```python
from build123d import *

# Parameters (mm, degrees)
SKETCH1_R                 = 9.8
BOSS_EXTRUDE1_DEPTH       = 15.7
FILLET1_R                 = 1
SKETCH3_W                 = 41.9
SKETCH3_H                 = 37
BOSS_EXTRUDE2_DEPTH       = 37.89
SKETCH2_R                 = 1.55
CUT_EXTRUDE1_DEPTH        = 61.440388814
SKETCH4_W                 = 4.95
SKETCH4_H                 = 37
BOSS_EXTRUDE3_DEPTH       = 14.25
CUT_EXTRUDE_START         = -14.25
CUT_EXTRUDE_2_OUTLINE_W   = 1.15
CUT_EXTRUDE_2_OUTLINE_H   = 14.2
CUT_EXTRUDE_2_OUTLINE_W_2 = 1.900000227
CUT_EXTRUDE_2_OUTLINE_H_2 = 18.6
CUT_EXTRUDE_2_DEPTH       = 14.25
CUT_EXTRUDE_1_REACH       = 83.854
SKETCH_1_R                = 1.05
CUT_EXTRUDE3_START        = -5
SKETCH6_R                 = 1.41
CUT_EXTRUDE3_DEPTH        = 69.371779997
FILLET5_R                 = 2
MOVE_START                = 11.2
MOVE_FACE_1_OUTLINE_R     = 9.8
MOVE_FACE_1_DEPTH         = 4.5
SKETCH_4_R                = 11.200313663
CUT_EXTRUDE_3_DEPTH       = 38.09
SKETCH_6_W                = 2.268388773
SKETCH_6_H                = 19.352707125
EXTRUDE_1_DEPTH           = 5
CUT_EXTRUDE2_REACH        = 83.854
SKETCH5_R                 = 1.05
SKETCH_7_W                = 33.485055755
SKETCH_7_H                = 15.84059592
EXTRUDE_2_DEPTH           = 5.9
SKETCH_8_W                = 34.098293505
SKETCH_8_H                = 15.557673108
EXTRUDE_3_DEPTH           = 5.9
OTHER_START               = 11.2
OTHER_1_DEPTH             = 42.39
SKETCH_9_R                = 3.5
CUT_EXTRUDE_4_DEPTH       = 5


# Read off the part's stored shape, not the designer's step: 切除-拉伸2, 移动面1, 填充阵列1
with BuildPart() as part:
    # Sketch1 → Boss-Extrude1 (new body)
    with BuildSketch(Plane(origin=(0, 0, 0), x_dir=(1, 0, 0), z_dir=(0, 1, 0))):
        with Locations(Location((0, 0, 0), (0, 0, 270))):
            Circle(SKETCH1_R)
    extrude(amount=BOSS_EXTRUDE1_DEPTH)

    # Fillet1
    fillet1_edges = [part.edges().sort_by_distance(p)[0] for p in [
        (0, 0, -9.8),
    ]]
    fillet(fillet1_edges, radius=FILLET1_R)

    # Sketch3 → Boss-Extrude2 (add)
    with BuildSketch(Plane(origin=(0, 15.7, 0), x_dir=(1, 0, 0), z_dir=(0, 1, 0))):
        Rectangle(SKETCH3_W, SKETCH3_H)
    extrude(amount=BOSS_EXTRUDE2_DEPTH)

    # Sketch2 → Cut-Extrude1 (cut, through all)
    with BuildSketch(Plane(origin=(0, 0, 0), x_dir=(-1, 0, 0), z_dir=(0, -1, 0))):
        with Locations(Location((0, 6.999998127, 0), (0, 0, 90))):
            Circle(SKETCH2_R)
        with Locations(Location((6.999998127, 0, 0), (0, 0, 90))):
            Circle(SKETCH2_R)
        with Locations(Location((0, -6.999998127, 0), (0, 0, 90))):
            Circle(SKETCH2_R)
        with Locations(Location((-6.999998127, 0, 0), (0, 0, 90))):
            Circle(SKETCH2_R)
    extrude(amount=-CUT_EXTRUDE1_DEPTH, mode=Mode.SUBTRACT)

    # Sketch4 → Boss-Extrude3 (add)
    with BuildSketch(Plane(origin=(0, 53.59, 0), x_dir=(1, 0, 0), z_dir=(0, 1, 0))):
        with Locations((-18.475, 0)):
            Rectangle(SKETCH4_W, SKETCH4_H)
        with Locations((18.475, 0)):
            Rectangle(SKETCH4_W, SKETCH4_H)
    extrude(amount=BOSS_EXTRUDE3_DEPTH)

    # 切除-拉伸2 outline → 切除-拉伸2 (cut)
    with BuildSketch(Plane(origin=(0, 67.84, 0), x_dir=(1, 0, 0), z_dir=(0, 1, 0)).offset(CUT_EXTRUDE_START)):
        with Locations((16.575, 0)):
            Rectangle(CUT_EXTRUDE_2_OUTLINE_W, CUT_EXTRUDE_2_OUTLINE_H)
        with Locations((-16.950000113, 0)):
            Rectangle(CUT_EXTRUDE_2_OUTLINE_W_2, CUT_EXTRUDE_2_OUTLINE_H_2)
    extrude(amount=CUT_EXTRUDE_2_DEPTH, mode=Mode.SUBTRACT)

    # 草图1 → 切除-拉伸1 (cut, up to next)
    with BuildSketch(Plane(origin=(20.95, 0, 0), x_dir=(0, 0, -1), z_dir=(1, 0, 0)), mode=Mode.PRIVATE) as cut_extrude_1_sk1:
        with Locations((-10.25, 59.7)):
            Circle(SKETCH_1_R)
    cut_extrude_1_tool1 = extrude(cut_extrude_1_sk1.sketch, amount=-CUT_EXTRUDE_1_REACH, mode=Mode.PRIVATE) & part.part
    # 草图1 → 切除-拉伸1 (cut, up to next)
    with BuildSketch(Plane(origin=(20.95, 0, 0), x_dir=(0, 0, -1), z_dir=(1, 0, 0)), mode=Mode.PRIVATE) as cut_extrude_1_sk2:
        with Locations((10.25, 59.7)):
            Circle(SKETCH_1_R)
    cut_extrude_1_tool2 = extrude(cut_extrude_1_sk2.sketch, amount=-CUT_EXTRUDE_1_REACH, mode=Mode.PRIVATE) & part.part
    add(cut_extrude_1_tool1.solids().sort_by_distance((20.95, 59.7, 10.25))[0], mode=Mode.SUBTRACT)
    add(cut_extrude_1_tool2.solids().sort_by_distance((20.95, 59.7, -10.25))[0], mode=Mode.SUBTRACT)

    # Sketch6 → Cut-Extrude3 (cut, through all)
    with BuildSketch(Plane.XZ.offset(CUT_EXTRUDE3_START)):
        with Locations((0, 6.999998127)):
            Circle(SKETCH6_R)
        with Locations((0, -6.999998127)):
            Circle(SKETCH6_R)
        with Locations((-6.999998127, 0)):
            Circle(SKETCH6_R)
        with Locations((6.999998127, 0)):
            Circle(SKETCH6_R)
    extrude(amount=-CUT_EXTRUDE3_DEPTH, mode=Mode.SUBTRACT)

    # Fillet5
    fillet5_edges = [part.edges().sort_by_distance(p)[0] for p in [
        (20.95, 41.77, -18.5),
        (-20.95, 41.77, -18.5),
        (-20.95, 41.77, 18.5),
        (20.95, 41.77, 18.5),
    ]]
    fillet(fillet5_edges, radius=FILLET5_R)

    # Move Face 1 outline → Move Face 1 (add)
    with BuildSketch(Plane(origin=(0, 0, 0), x_dir=(1, 0, 0), z_dir=(0, 1, 0)).offset(MOVE_START)):
        with BuildLine():
            Line((20.95, -16.5), (20.95, 16.5))
            ThreePointArc((20.95, 16.5), (20.364213562, 17.914213562), (18.95, 18.5))
            Line((18.95, 18.5), (-18.95, 18.5))
            ThreePointArc((-18.95, 18.5), (-20.364213562, 17.914213562), (-20.95, 16.5))
            Line((-20.95, 16.5), (-20.95, -16.5))
            ThreePointArc((-20.95, -16.5), (-20.364213562, -17.914213562), (-18.95, -18.5))
            Line((-18.95, -18.5), (18.95, -18.5))
            ThreePointArc((18.95, -18.5), (20.364213562, -17.914213562), (20.95, -16.5))
        make_face()
        Circle(MOVE_FACE_1_OUTLINE_R, mode=Mode.SUBTRACT)
    extrude(amount=MOVE_FACE_1_DEPTH)

    # 草图4 → 切除-拉伸3 (cut)
    with BuildSketch(Plane(origin=(0, 53.59, 0), x_dir=(1, 0, 0), z_dir=(0, 1, 0))):
        with Locations(Location((0, 0, 0), (0, 0, 270))):
            Circle(SKETCH_4_R)
    extrude(amount=-CUT_EXTRUDE_3_DEPTH, mode=Mode.SUBTRACT)

    # 草图6 → 凸台-拉伸1 (add)
    with BuildSketch(Plane(origin=(0, 53.59, 0), x_dir=(1, 0, 0), z_dir=(0, 1, 0))):
        with Locations((-17.13419541, 0.070716348)):
            Rectangle(SKETCH_6_W, SKETCH_6_H)
    extrude(amount=EXTRUDE_1_DEPTH)

    # Sketch5 → Cut-Extrude2 (cut, up to next)
    with BuildSketch(Plane.ZY.offset(20.95), mode=Mode.PRIVATE) as cut_extrude2_sk1:
        with Locations((-10.25, 55.95)):
            Circle(SKETCH5_R)
    cut_extrude2_tool1 = extrude(cut_extrude2_sk1.sketch, amount=-CUT_EXTRUDE2_REACH, mode=Mode.PRIVATE) & part.part
    # Sketch5 → Cut-Extrude2 (cut, up to next)
    with BuildSketch(Plane.ZY.offset(20.95), mode=Mode.PRIVATE) as cut_extrude2_sk2:
        with Locations((10.25, 55.95)):
            Circle(SKETCH5_R)
    cut_extrude2_tool2 = extrude(cut_extrude2_sk2.sketch, amount=-CUT_EXTRUDE2_REACH, mode=Mode.PRIVATE) & part.part
    add(cut_extrude2_tool1.solids().sort_by_distance((-20.95, 55.95, -10.25))[0], mode=Mode.SUBTRACT)
    add(cut_extrude2_tool2.solids().sort_by_distance((-20.95, 55.95, 10.25))[0], mode=Mode.SUBTRACT)

    # 草图7 → 凸台-拉伸2 (add)
    with BuildSketch(Plane.XY.offset(18.5)):
        with Locations((0.159698038, 59.91970204)):
            Rectangle(SKETCH_7_W, SKETCH_7_H)
    extrude(amount=-EXTRUDE_2_DEPTH)

    # 草图8 → 凸台-拉伸3 (add)
    with BuildSketch(Plane(origin=(0, 0, -18.5), x_dir=(-1, 0, 0), z_dir=(0, 0, -1))):
        with Locations((-0.100853247, 60.061163446)):
            Rectangle(SKETCH_8_W, SKETCH_8_H)
    extrude(amount=-EXTRUDE_3_DEPTH)

    # Other 1 outline → Other 1 (cut)
    with BuildSketch(Plane(origin=(0, 0, 0), x_dir=(1, 0, 0), z_dir=(0, 1, 0)).offset(OTHER_START)):
        Polygon((15.149306373, -4.606205589), (16.015331777, -4.106205589), (16.015331777, -3.106205589), (15.149306373, -2.606205589), (14.283280969, -3.106205589), (14.283280969, -4.106205589), align=None)
        Polygon((16.015331777, 3.106205589), (16.015331777, 4.106205589), (15.149306373, 4.606205589), (14.283280969, 4.106205589), (14.283280969, 3.106205589), (15.149306373, 2.606205589), align=None)
        Polygon((-11.917262605, 6.212411178), (-11.051237202, 6.712411178), (-11.051237202, 7.712411178), (-11.917262605, 8.212411178), (-12.783288009, 7.712411178), (-12.783288009, 6.712411178), align=None)
        Polygon((-11.051237202, -7.712411178), (-11.051237202, -6.712411178), (-11.917262605, -6.212411178), (-12.783288009, -6.712411178), (-12.783288009, -7.712411178), (-11.917262605, -8.212411178), align=None)
        Polygon((13.933288009, -6.712411178), (13.067262605, -6.212411178), (12.201237202, -6.712411178), (12.201237202, -7.712411178), (13.067262605, -8.212411178), (13.933288009, -7.712411178), align=None)
        Polygon((13.933288009, -0.5), (13.933288009, 0.5), (13.067262605, 1), (12.201237202, 0.5), (12.201237202, -0.5), (13.067262605, -1), align=None)
        Polygon((13.933288009, 6.712411178), (13.933288009, 7.712411178), (13.067262605, 8.212411178), (12.201237202, 7.712411178), (12.201237202, 6.712411178), (13.067262605, 6.212411178), align=None)
        Polygon((-13.999306373, 2.606205589), (-13.133280969, 3.106205589), (-13.133280969, 4.106205589), (-13.999306373, 4.606205589), (-14.865331777, 4.106205589), (-14.865331777, 3.106205589), align=None)
        Polygon((-13.133280969, -4.106205589), (-13.133280969, -3.106205589), (-13.999306373, -2.606205589), (-14.865331777, -3.106205589), (-14.865331777, -4.106205589), (-13.999306373, -4.606205589), align=None)
    extrude(amount=OTHER_1_DEPTH, mode=Mode.SUBTRACT)

    # 草图9 → 切除-拉伸4 (cut)
    with BuildSketch(Plane.XZ):
        with Locations(Location((0, 0, 0), (0, 0, 270))):
            Circle(SKETCH_9_R)
    extrude(amount=-CUT_EXTRUDE_4_DEPTH, mode=Mode.SUBTRACT)


solid = part.part
```
Check sheet for the modelled part. Datum: model origin and axes. Units: mm. A direction names the side the tool comes from. Coordinates: 2 decimals unless noted, no trailing zeros. Write each loop counter-clockwise with the first axis right and the second up, starting at its lowest first coordinate (ties: lowest second). Pieces come first, ordered by that corner, then holes. Notation, with made-up numbers: (15.25, 77.25) -> (51.25, 77.25) arc R12 ccw to (51.25, 86.25) -> close; hole circle Ø3 at (-18, 56.5). An arc over 180 degrees is marked (long way). Use a Markdown table: item, result.
1. Go/stop test with flat-tipped pins: pin 1 Ø5 at (x, z) = (-10.5, 0) entering from +Y; pin 2 Ø11 at (x, z) = (-1, -1) entering from +Y. Record where each tip stops, or that it passes through.
Reported:
| item | result |
|---|---|
| pin 1 | stops at y = 53.59 |
| pin 2 | stops at y = 15.5 |
2. Sectioned sample at A-A (y = 22.5). Give the number of separate pieces and of enclosed holes in the cut face, plus the area to 3 significant figures.
Reported:
| item | result |
|---|---|
| separate pieces | 1 |
| enclosed holes | 10 |
| area | 1,130 mm2 |
3. Tool access check on faces 1 (the flat face through (9, 11.2, -4.4)), 2 (the cylindrical face through (-18.5, 55, 10.7)), 3 (the flat face through (0, 61, -12.6)). Record the directions out of +Z, -Z, +X, -X, +Y, -Y that give a thin tool (end or side, any length) a straight path to the whole face; none if there is none.
Reported:
| item | result |
|---|---|
| face 1 | -Y |
| face 2 | -X |
| face 3 | +Y |
4. Scan lines: line 1 along X through (y, z) = (42, 0); line 2 along Y through (x, z) = (-18.05, 10.25); line 3 along Z through (x, y) = (-3, 54.5). Record each from-to range of solid material in increasing order.
Reported:
| item | result |
|---|---|
| line 1 | x = -20.95 to -11.2, 11.2 to 12.2, 13.93 to 20.95 |
| line 2 | y = 11.2 to 54.9, 57 to 67.84 |
| line 3 | z = -18.5 to -12.6, 12.6 to 18.5 |
5. Sectioned sample at B-B (z = 15.5). Enter the section's corners in (x, y).
Reported:
| item | result |
|---|---|
| outline | (-20.95, 11.2) -> (20.95, 11.2) -> (20.95, 67.84) -> (-20.95, 67.84) -> close |
6. Release check for a two-part mould opening along X. For faces 4 (the flat face through (16, 61, -9)), 5 (the cylindrical face through (2.94, 6.03, 9.35)), 6 (the cylindrical face through (20.35, 39.12, 17.93)) record: pulls with the +X half, pulls with the -X half, needs draft (parallel to the pull), parting line crosses it, or undercut.
Reported:
| item | result |
|---|---|
| face 4 | undercut |
| face 5 | parting line crosses it |
| face 6 | pulls with the +X half |
